from build123d import *

# Parameters (mm, degrees)
SKETCH1_R           = 3
BOSS_EXTRUDE1_DEPTH = 12
SKETCH2_W           = 5.91565448
SKETCH2_H           = 1.002512874
BOSS_EXTRUDE2_DEPTH = 10
SKETCH4_R           = 2
BOSS_EXTRUDE3_DEPTH = 7.5


with BuildPart() as part:
    # Sketch1 → Boss-Extrude1 (new body)
    with BuildSketch(Plane.XY):
        Circle(SKETCH1_R)
    extrude(amount=BOSS_EXTRUDE1_DEPTH)

    # Sketch2 → Boss-Extrude2 (add)
    with BuildSketch(Plane(origin=(0, 0, 0), x_dir=(-1, 0, 0), z_dir=(0, 0, -1))):
        Rectangle(SKETCH2_W, SKETCH2_H)
    extrude(amount=BOSS_EXTRUDE2_DEPTH)

    # Sketch4 → Boss-Extrude3 (add)
    with BuildSketch(Plane(origin=(0, 0.501256437, 0), x_dir=(1, 0, 0), z_dir=(0, 1, 0))):
        with Locations((0, 7)):
            Circle(SKETCH4_R)
    extrude(amount=BOSS_EXTRUDE3_DEPTH)


solid = part.part
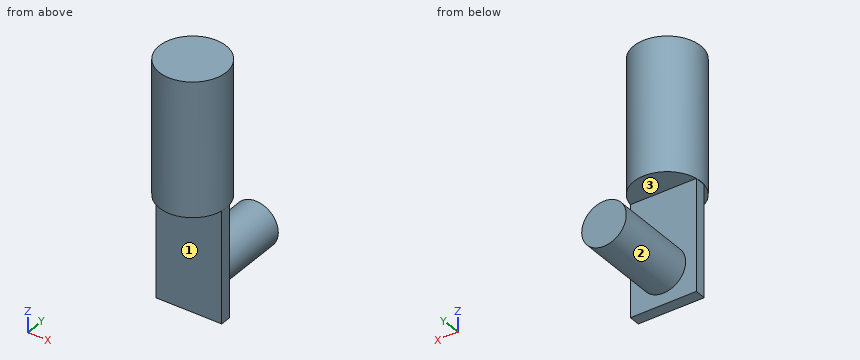
Verification items for the finished model (mm, model axes). Face numbers are marked on the shaded views. A direction names the side the tool comes from. Round coordinates to 2 decimals unless told otherwise and drop trailing zeros. Loops run counter-clockwise (first coordinate to the right, second up) from the corner with the lowest first, then second, coordinate; pieces in that order, holes last. Notation, with made-up numbers: (21, -35.5) - (36, -35.5) arc R24 ccw to (36, -6.5) - close; hole circle Ø5 at (45, 56). An arc over 180 degrees is marked (long way). Use one line per item in the form item = value.
1. Section check D-D on x = -0.9. Record the cut outline in (y, z), and give its area (3 significant figures).
A:
outline = (-2.86, 0) - (-0.5, 0) - (-0.5, -10) - (0.5, -10) - (0.5, -8.79) - (8, -8.79) - (8, -5.21) - (0.5, -5.21) - (0.5, 0) - (2.86, 0) - (2.86, 12) - (-2.86, 12) - close
area = 105 mm²
2. Section check B-B on z = 3. Record the cut outline in (x, y), and give its area (3 significant figures).
A:
outline = circle Ø6 at (0, 0)
area = 28.3 mm²
3. Section check A-A on x = 0. Record the cut outline in (y, z).
A:
outline = (-3, 0) - (-0.5, 0) - (-0.5, -10) - (0.5, -10) - (0.5, -9) - (8, -9) - (8, -5) - (0.5, -5) - (0.5, 0) - (3, 0) - (3, 12) - (-3, 12) - close
4. Scan lines: probe 1 along Z at (x, y) = (0.65, -1); probe 2 along Y at (x, z) = (-1.9, -3); probe 3 along Z at (x, y) = (0.4, 2.25). Record each from-to range of solid material in increasing order.
A:
probe_1 = 0 to 12
probe_2 = -0.5 to 0.5
probe_3 = -8.96 to -5.04, 0 to 12
5. Section check C-C on y = 4. Record the cut outline in (x, z), and give its area (3 significant figures).
A:
outline = circle Ø4 at (0, -7)
area = 12.6 mm²
6. Access from +Z, -Z, +X, -X, +Y, -Y to the whole of each face (thin tool, end or side, straight path). Record for the marked faces 1, 2 and 3.
A:
face_1 = -Z, +X, -X, -Y
face_2 = +Y
face_3 = +X, -X, +Y
7. Gauge pin test, flat ends, axial feed: pin 1 Ø1.8 at (x, z) = (-1.5, -3.5) entering from +Y; pin 2 Ø1.2 at (x, y) = (-0.5, -1.5) entering from -Z; pin 3 Ø1 at (x, z) = (-2, 0) entering from +Y. Record the tip position at first contact, or that the pin passes through.
A:
pin_1 = 0.5
pin_2 = 0
pin_3 = 2.6
